Could you check a few things on this model? Use its own coordinates, in mm. A direction names the side the tool comes from. Coordinates: 2 decimals unless noted, no trailing zeros. Order: outer loops, then holes, each group sorted by start corner. A loop starts at its lowest first (then second) coordinate and runs counter-clockwise, first axis right, second up. Notation, with made-up numbers: (56.25, 74.5) - (89.25, 74.5) arc R13 ccw to (89.25, 95.5) - close; hole circle Ø8 at (7.5, 59.5). An arc over 180 degrees is marked (long way). Answer as a JSON object with one key per item and string values. Group by question number.
(1) Will these pins go through, and if not, where does the flat tip stop? P1, Ø13, axis at x = 71.5, y = 44, coming from the +Z side; P2, Ø2.5, axis at x = 18.5, y = 3.5, coming from the -Z side; P3, Ø2, axis at x = 4, y = 90, coming from the -Z side.
(2) Which directions (+Z, -Z, +X, -X, +Y, -Y) give clear straight access to the entire face, cutting with the end or side of a thin tool? Please do faces 1 (the cylindrical face through (62.013, 39.772, 6.521)), 2 (the flat face through (5, 11, 2.184)), 3 (the cylindrical face through (65.01, 39.64, 2.54)).
(3) Imagine slicing it at A-A, the plane y = 39.2. Write out the boundary of the cut face in (x, z), and give its area (3 significant figures).
(4) We'd pull the mould along Y, two halves only. Please class faces 4 (the flat face through (133, 5, 2.184)), 5 (the flat face through (150, 49, 4)), 6 (the flat face through (74, 0, 4)): pulls with the +Y half, pulls with the -Y half, needs draft (parallel to the pull), parting line crosses it, or undercut.
(5) Imagine slicing it at B-B, the plane z = 6.25. Give the number of separate pieces and of enclosed holes in the cut face, and give its area (3 significant figures).
(6) Please list where these lines run through material, in increasing order: probe 1 along Y at (x, z) = (146, 1.15); probe 2 along Y at (x, z) = (146, 5.75); probe 3 along X at (y, z) = (94.5, 4).
from build123d import *

# Parameters (mm, degrees)
SKETCH1_W                                      = 150
SKETCH1_H                                      = 100
BOSS_EXTRUDE1_DEPTH                            = 8
CBORE_FOR_2_SOCKET_HEAD_CAP_SCREW1_D           = 2.4384
CBORE_FOR_2_SOCKET_HEAD_CAP_SCREW1_CBORE_D     = 4.7625
CBORE_FOR_2_SOCKET_HEAD_CAP_SCREW1_CBORE_DEPTH = 2.1844
SKETCH5_R                                      = 10
CUT_EXTRUDE1_DEPTH                             = 9
SKETCH6_R                                      = 13
CUT_EXTRUDE2_DEPTH                             = 3
F_2_56_TAPPED_HOLE1_D                          = 1.778
F_2_56_TAPPED_HOLE1_DEPTH                      = 15
F_2_56_TAPPED_HOLE1_TIP                        = 0.53416509


with BuildPart() as part:
    # Sketch1 → Boss-Extrude1 (new body)
    with BuildSketch(Plane.XY):
        with Locations((75, 50)):
            Rectangle(SKETCH1_W, SKETCH1_H)
    extrude(amount=BOSS_EXTRUDE1_DEPTH)

    # CBORE for #2 Socket Head Cap Screw1 (through all)
    with Locations(Plane(origin=(0, 0, 0), x_dir=(-1, 0, 0), z_dir=(0, 0, -1))):
        with Locations((-132, 4), (-18, 4), (-4, 90), (-146, 90), (-146, 10), (-4, 10), (-75, 4)):
            CounterBoreHole(CBORE_FOR_2_SOCKET_HEAD_CAP_SCREW1_D / 2, CBORE_FOR_2_SOCKET_HEAD_CAP_SCREW1_CBORE_D / 2, CBORE_FOR_2_SOCKET_HEAD_CAP_SCREW1_CBORE_DEPTH)

    # Sketch5 → Cut-Extrude1 (cut, through all)
    with BuildSketch(Plane.XY.offset(8)):
        with Locations((75, 39.2)):
            Circle(SKETCH5_R)
    extrude(amount=-CUT_EXTRUDE1_DEPTH, mode=Mode.SUBTRACT)

    # Sketch6 → Cut-Extrude2 (cut)
    with BuildSketch(Plane.XY.offset(8)):
        with Locations((75, 39.2)):
            Circle(SKETCH6_R)
    extrude(amount=-CUT_EXTRUDE2_DEPTH, mode=Mode.SUBTRACT)

    # #2-56 Tapped Hole1
    with Locations(Plane(origin=(0, 100, 0), x_dir=(1, 0, 0), z_dir=(0, 1, 0))):
        with Locations((18, -4), (75, -4), (132, -4)):
            Hole(F_2_56_TAPPED_HOLE1_D / 2, depth=F_2_56_TAPPED_HOLE1_DEPTH)
            with Locations((0, 0, -(F_2_56_TAPPED_HOLE1_DEPTH + F_2_56_TAPPED_HOLE1_TIP / 2))):  # 118° drill point
                Cone(0, F_2_56_TAPPED_HOLE1_D / 2, F_2_56_TAPPED_HOLE1_TIP, mode=Mode.SUBTRACT)


solid = part.part
Result set:
{
 "1": {"P1": "stops at z = 5", "P2": "stops at z = 2.18", "P3": "passes through"},
 "2": {"face 1": "+Z", "face 2": "-Z", "face 3": "+Z, -Z"},
 "3": {"outline": "(0, 0) - (65, 0) - (65, 5) - (62, 5) - (62, 8) - (0, 8) - close; (85, 0) - (150, 0) - (150, 8) - (88, 8) - (88, 5) - (85, 5) - close", "area": "1,020 mm^2"},
 "4": {"face 4": "undercut", "face 5": "needs draft", "face 6": "pulls with the -Y half"},
 "5": {"separate pieces": "1", "enclosed holes": "8", "area": "14,400 mm^2"},
 "6": {"probe 1": "y = 0 to 7.62, 12.38 to 87.62, 92.38 to 100", "probe 2": "y = 0 to 8.78, 11.22 to 88.78, 91.22 to 100", "probe 3": "x = 0 to 17.11, 18.89 to 74.11, 75.89 to 131.11, 132.89 to 150"}
}
